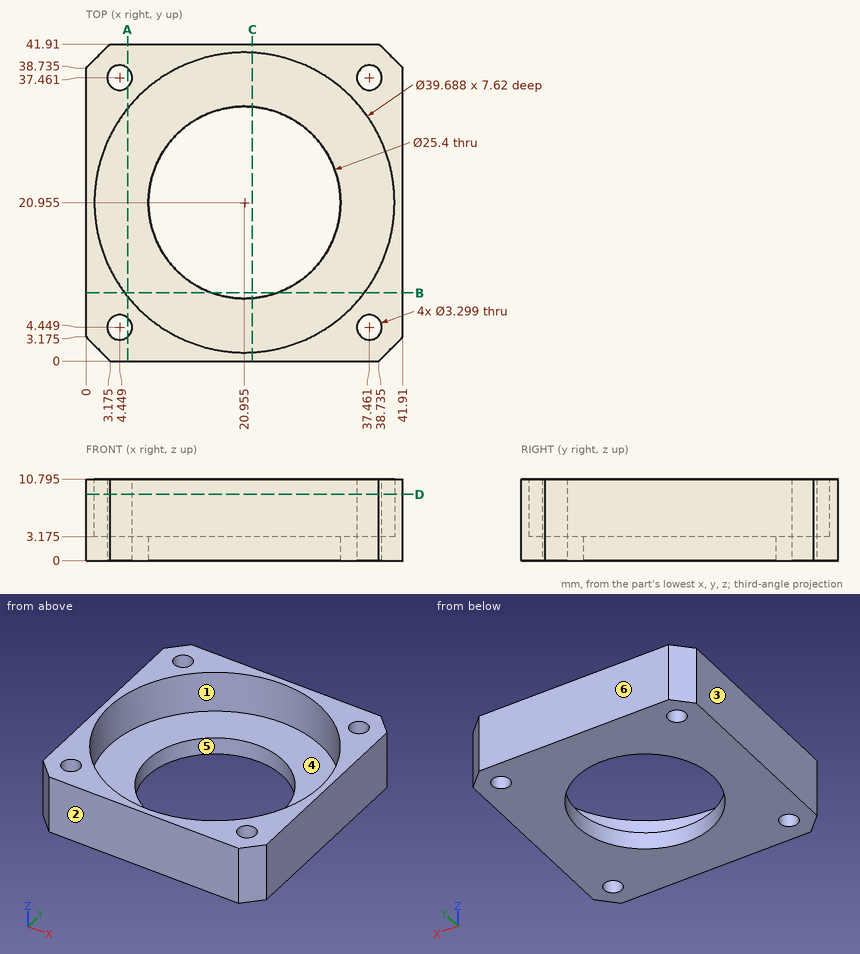
Study the drawing (mm; zero at the part's minimum x, y, z) and answer. A direction names the side the tool comes from. Round coordinates to 2 decimals unless told otherwise and drop trailing zeros. Write each loop counter-clockwise with the first axis right and the second up, starting at its lowest first coordinate (ties: lowest second). Pieces come first, ordered by that corner, then holes. Notation, with made-up numbers: (-24, 58.5) -> (22, 58.5) arc R14 ccw to (22, 66.5) -> close; hole circle Ø10 at (-33.75, -33). An arc over 180 degrees is marked (long way). Write each question's results on one line, items separated by ' | '.
Item 1: Which of the six approach directions +Z, -Z, +X, -X, +Y, -Y give full straight-line access (tool end or side, diameter ignored) to the marked faces 1 and 2?
Result set:
face 1: +Z | face 2: +Z, -Z, +X, -X, -Y
Item 2: The mould has two halves that part along Y. Classify the marked faces 3, 4, 5 and 6: +Y half, -Y half, draft (parallel to the pull), parting line (faces both ways), or undercut.
Result set:
face 3: draft | face 4: undercut | face 5: undercut | face 6: +Y half
Item 3: Find the intervals of material crossed by line 1 along Y through (x, z) = (21, 10.25); line 2 along Y through (x, z) = (5, 9.5) (1 decimal); line 3 along X through (y, z) = (18, 8), in increasing order. Write a range as [from, to].
Result set:
line 1: [0, 1.11], [40.8, 41.91] | line 2: [0, 2.9], [6, 9.2], [32.8, 35.9], [39, 41.9] | line 3: [0, 1.33], [40.58, 41.91]
Item 4: A cutting plane is placed at B-B, the plane y = 9. Determine the outline of the cut face in (x, z) (1 decimal).
Result set:
outline: (0, 0) -> (16.7, 0) -> (16.7, 3.2) -> (5.1, 3.2) -> (5.1, 10.8) -> (0, 10.8) -> close; (25.2, 0) -> (41.9, 0) -> (41.9, 10.8) -> (36.8, 10.8) -> (36.8, 3.2) -> (25.2, 3.2) -> close
Item 5: A cutting plane is placed at A-A, the plane x = 5.5. Determine the outline of the cut face in (y, z) (1 decimal), plus the area to 3 significant figures.
Result set:
outline: (0, 0) -> (3.2, 0) -> (3.2, 10.8) -> (0, 10.8) -> close; (5.7, 0) -> (36.2, 0) -> (36.2, 10.8) -> (33.4, 10.8) -> (33.4, 3.2) -> (8.5, 3.2) -> (8.5, 10.8) -> (5.7, 10.8) -> close; (38.7, 0) -> (41.9, 0) -> (41.9, 10.8) -> (38.7, 10.8) -> close | area: 208 mm^2
Item 6: A cutting plane is placed at C-C, the plane x = 22. Determine the outline of the cut face in (y, z) (1 decimal).
Result set:
outline: (0, 0) -> (8.3, 0) -> (8.3, 3.2) -> (1.1, 3.2) -> (1.1, 10.8) -> (0, 10.8) -> close; (33.6, 0) -> (41.9, 0) -> (41.9, 10.8) -> (40.8, 10.8) -> (40.8, 3.2) -> (33.6, 3.2) -> close
Item 7: A cutting plane is placed at D-D, the plane z = 8.75. Count the separate pieces of the cut face and the enclosed holes in it, plus the area to 3 significant figures.
Result set:
separate pieces: 1 | enclosed holes: 5 | area: 465 mm^2
Item 8: A flat-ended cylindrical pin translates along its axis: P1, Ø3, axis at x = 30.5, y = 28.5, coming from the +Z side (1 decimal). Find the tip coordinate at first contact, or state that the pin passes through.
Result set:
P1: z = 3.2
